Could you check a few things on this model? Use its own coordinates, in mm. A direction names the side the tool comes from. Round coordinates to 2 decimals unless told otherwise and drop trailing zeros. Write each loop counter-clockwise with the first axis right and the second up, starting at its lowest first coordinate (ties: lowest second). Pieces come first, ordered by that corner, then holes. Notation, with made-up numbers: (7, 16.25) - (59, 16.25) arc R17 ccw to (59, 26.25) - close; hole circle Ø2 at (78.5, 4.5). An arc over 180 degrees is marked (long way). Write each question's results on one line, items separated by ' | '. Start each with the question number.
(1) Imagine slicing it at C-C on y = 4. Write out the boundary of the cut face in (x, z), then the cut area to 3 significant figures.
(2) Please list where these lines run through material, in increasing order: line 1 (Z direction, x = -2.25, y = -1.5); line 2 (Z direction, x = -3.25, y = 0.25); line 3 (Z direction, x = -0.5, y = -4). Write a range as [from, to].
(3) Imagine slicing it at A-A on z = 9. Write out the boundary of the cut face in (x, y) (1 decimal).
(4) On a 3-axis mill with a long thin cutter (end or side, diameter ignored), from which of +Z, -Z, +X, -X, +Y, -Y can I reach the whole of each face in a straight line? I mean faces 1 (the cylindrical face through (0.85, -1.634, 36.826)), 2 (the flat face through (0, 0, 37.084)). Say none if no direction works.
(5) Imagine slicing it at B-B on x = 3.75. Write out the boundary of the cut face in (y, z).
(6) For P1, Ø6, axis at y = 2, z = 10.5, coming from the -X side; P2, Ø6, axis at x = -2, z = 33, coming from the -Y side; P3, Ø4, axis at x = 0.5, z = 18, coming from the +Y side, each with a flat end and sliding along its axis, tell me the tip position at first contact or that it passes through.
```python
from build123d import *

# Parameters (mm, degrees)
SKETCH3_R           = 3.175
BOSS_EXTRUDE1_DEPTH = 3.556
CUT_SWEEP1_PITCH    = 1.27
SKETCH10_R          = 2.2225
BOSS_EXTRUDE5_DEPTH = 33.02
SKETCH9_R           = 5.08
BOSS_EXTRUDE4_DEPTH = 0.127
DOME3_FACE_RADIUS   = 5.08
DOME3_HEIGHT        = 2.38
SKETCH11_R          = 1.8415
BOSS_EXTRUDE6_DEPTH = 0.508


with BuildPart() as part:
    # Sketch3 → Boss-Extrude1 (new body)
    with BuildSketch(Plane.XY):
        Circle(SKETCH3_R)
    extrude(amount=BOSS_EXTRUDE1_DEPTH)

    # Cut-Sweep1: arcs per turn and ends read off the stored shape
    # Cut-Sweep1: the profile of Sketch5 profile screwed along a left-hand helix through 5 turns, 8 arcs to a turn; built about Z, then put on its axis
    cut_sweep1_z = Axis((0, 0, 0), (0, 0, 1))
    cut_sweep1_corners = [(2.54, 0, -1.397), (3.1753, 0, -1.763790626), (3.1753, 0, -0.776209374), (2.54, 0, -1.143)]
    with BuildLine(mode=Mode.PRIVATE) as cut_sweep1_profile:
        Line(cut_sweep1_corners[0], cut_sweep1_corners[1])
        Line(cut_sweep1_corners[1], cut_sweep1_corners[2])
        Line(cut_sweep1_corners[2], cut_sweep1_corners[3])
        Line(cut_sweep1_corners[3], cut_sweep1_corners[0])
    cut_sweep1_cap = Face(cut_sweep1_profile.wire())
    cut_sweep1_turn_angles = [0, -22.5, -45, -67.5, -90, -112.5, -135, -157.5, -180, -202.5, -225, -247.5, -270, -292.5, -315, -337.5, -360]
    cut_sweep1_turn_weights = [1, 0.9238795325112867, 1, 0.9238795325112867, 1, 0.9238795325112867, 1, 0.9238795325112867, 1, 0.9238795325112867, 1, 0.9238795325112867, 1, 0.9238795325112867, 1, 0.9238795325112867, 1]
    cut_sweep1_turn_rails = [Edge.make_bspline([Vector(p[0], p[1], 0).rotate(cut_sweep1_z, cut_sweep1_turn_angles[k]) / cut_sweep1_turn_weights[k] + Vector(0, 0, p[2] + -CUT_SWEEP1_PITCH * cut_sweep1_turn_angles[k] / 360) for k in range(17)], [0, 0, 0, 1, 1, 2, 2, 3, 3, 4, 4, 5, 5, 6, 6, 7, 7, 8, 8, 8], 2, cut_sweep1_turn_weights) for p in cut_sweep1_corners]
    cut_sweep1_turn_sides = [Face.make_surface_from_curves(cut_sweep1_turn_rails[p[0]], cut_sweep1_turn_rails[p[1]]) for p in [(0, 1), (1, 2), (2, 3), (3, 0)]]
    cut_sweep1 = Plane(origin=(0, 0, 0), x_dir=(0, 1, 0), z_dir=(0, 0, 1)) * Solid(Shell([*[p.moved(Location((0, 0, CUT_SWEEP1_PITCH * i))) for i in range(5) for p in cut_sweep1_turn_sides], cut_sweep1_cap, cut_sweep1_cap.rotate(cut_sweep1_z, -1800).moved(Location((0, 0, -CUT_SWEEP1_PITCH * -1800 / 360)))]))
    add(cut_sweep1, mode=Mode.SUBTRACT)

    # Sketch10 → Boss-Extrude5 (add)
    with BuildSketch(Plane.XY.offset(3.556)):
        Circle(SKETCH10_R)
    extrude(amount=BOSS_EXTRUDE5_DEPTH)

    # Sketch9 → Boss-Extrude4 (add)
    with BuildSketch(Plane.XY):
        Circle(SKETCH9_R)
    extrude(amount=-BOSS_EXTRUDE4_DEPTH)

    # Dome3: a dome of height H over a round flat face of radius A is a cap of a sphere of radius (A * A + H * H) / (2 * H)
    dome3_r = (DOME3_FACE_RADIUS * DOME3_FACE_RADIUS + DOME3_HEIGHT * DOME3_HEIGHT) / (2 * DOME3_HEIGHT)
    dome3_base = Plane((0, 0, -0.127), z_dir=(0, 0, -1))
    with Locations(dome3_base.offset(DOME3_HEIGHT - dome3_r)):
        dome3_ball = Sphere(dome3_r, mode=Mode.PRIVATE)
    add(split(dome3_ball, bisect_by=dome3_base, keep=Keep.TOP, mode=Mode.PRIVATE))

    # Sketch11 → Boss-Extrude6 (add)
    with BuildSketch(Plane.XY.offset(36.576)):
        Circle(SKETCH11_R)
    extrude(amount=BOSS_EXTRUDE6_DEPTH)


solid = part.part
```
Response:
1) outline: (-3.13, -0.13) arc R5.26 ccw to (3.13, -0.13) - (3.13, 0) - (-3.13, 0) - close | area: 5.20 mm²
2) line 1: [-1.93, 0.61], [1.05, 1.88], [2.32, 3.15] | line 2: [-1.65, 0] | line 3: [-1.14, 0]
3) outline: circle Ø4.4 at (0, 0)
4) face 1: +Z | face 2: +Z, +X, -X, +Y, -Y
5) outline: (-3.43, -0.13) arc R5.45 ccw to (3.43, -0.13) - (3.43, 0) - (-3.43, 0) - close
6) P1: x = -2.22 | P2: y = -2.22 | P3: y = 2.22
